```python
from build123d import *

# Parameters (mm, degrees)
SKICA1_R                 = 1.75
P_IDAT_VYSUNUT_M1_DEPTH  = 10
SKICA2_R                 = 6
ODEBRAT_VYSUNUT_M1_DEPTH = 6


with BuildPart() as part:
    # Skica1 → Přidat vysunutím1 (new body)
    with BuildSketch(Plane.XY):
        Polygon((25.815994553, 2.492123403), (25.815994553, 8.277058671), (19.815994553, 8.277058671), (19.815994553, 2.492123403), (19.815994553, -9.506219408), (19.815994553, -15.291154677), (25.815994553, -15.291154677), (25.815994553, -9.506219408), align=None)
        with Locations((22.815994553, -12.398687042)):
            Circle(SKICA1_R, mode=Mode.SUBTRACT)
        with Locations((22.815994553, 5.384591037)):
            Circle(SKICA1_R, mode=Mode.SUBTRACT)
    extrude(amount=P_IDAT_VYSUNUT_M1_DEPTH)

    # Skica2 → Odebrat vysunutím1 (cut)
    with BuildSketch(Plane.ZY.offset(-19.815994553)):
        with Locations((-0.099711825, -3.507048003)):
            Circle(SKICA2_R)
    extrude(amount=-ODEBRAT_VYSUNUT_M1_DEPTH, mode=Mode.SUBTRACT)


solid = part.part
```
Model file for the job. Use its own axes, mm. Round coordinates to 2 decimals unless told otherwise and drop trailing zeros. Order: outer loops, then holes, each group sorted by start corner. A loop starts at its lowest first (then second) coordinate and runs counter-clockwise, first axis right, second up. Notation, with made-up numbers: (66, 36) -> (91, 36) arc R21 ccw to (91, 62) -> close; hole circle Ø7 at (5, 25.5). An arc over 180 degrees is marked (long way). Use one line per item in the form item = value.
Item 1: Cut at B-B, the plane y = -12.75. Write the cut outline in (x, z), and give its area (3 significant figures).
Returned:
outline = (19.82, 0) -> (21.1, 0) -> (21.1, 10) -> (19.82, 10) -> close; (24.53, 0) -> (25.82, 0) -> (25.82, 10) -> (24.53, 10) -> close
area = 25.7 mm^2
Item 2: Flat gauge pins, fed straight in: pin 1 Ø3 at (x, y) = (22.82, 5.38) entering from +Z; pin 2 Ø1.5 at (x, y) = (24.5, -6) entering from -Z; pin 3 Ø3 at (y, z) = (-7, 4) entering from -X. Where does each tip first touch, or does it go through?
Returned:
pin_1 = through
pin_2 = 4.95
pin_3 = 19.82
Item 3: Pull direction Y, two halves, no side cores. Call faces 1 (the face through (19.816, -3, 7)), 2 (the face through (22.8, -3.6, 5.9)), 3 (the face through (23, 8.277, 5)): released by +Y, released by -Y, zero draft, split by the parting line, or undercut.
Returned:
face_1 = zero draft
face_2 = undercut
face_3 = released by +Y
Item 4: Cut at A-A, the plane z = 1.5. Write the cut outline in (x, y).
Returned:
outline = (19.82, -15.29) -> (25.82, -15.29) -> (25.82, -9.29) -> (19.82, -9.29) -> close; (19.82, 2.28) -> (25.82, 2.28) -> (25.82, 8.28) -> (19.82, 8.28) -> close; hole circle Ø3.5 at (22.82, -12.4); hole circle Ø3.5 at (22.82, 5.38)
Item 5: Cut at D-D, the plane z = 4. Write the cut outline in (x, y).
Returned:
outline = (19.82, -15.29) -> (25.82, -15.29) -> (25.82, -7.89) -> (19.82, -7.89) -> close; (19.82, 0.87) -> (25.82, 0.87) -> (25.82, 8.28) -> (19.82, 8.28) -> close; hole circle Ø3.5 at (22.82, -12.4); hole circle Ø3.5 at (22.82, 5.38)
Item 6: Drill centre lines: line 1 (Y direction, x = 24.15, z = 3); line 2 (Y direction, x = 23.65, z = 8.5); line 3 (Y direction, x = 22.45, z = 3.75). Where is each one in solid material? Low to high.
Returned:
line_1 = -15.29 to -13.53, -11.27 to -8.64, 1.63 to 4.25, 6.52 to 8.28
line_2 = -15.29 to -13.94, -10.86 to 3.85, 6.92 to 8.28
line_3 = -15.29 to -14.11, -10.69 to -8.11, 1.1 to 3.67, 7.1 to 8.28
Item 7: Cut at C-C, the plane x = 22.3. Write the cut outline in (y, z), and give its area (3 significant figures).
Returned:
outline = (-15.29, 0) -> (-14.07, 0) -> (-14.07, 10) -> (-15.29, 10) -> close; (-10.73, 0) -> (-9.51, 0) arc R6 cw to (2.49, 0) -> (3.71, 0) -> (3.71, 10) -> (-10.73, 10) -> close; (7.06, 0) -> (8.28, 0) -> (8.28, 10) -> (7.06, 10) -> close
area = 113 mm^2
